Autodesk Inventor part; units mm, degrees
ref_plane "to_ring_F_R_XY" through (20.575, 0, 0) normal (1, 0, 0) x (0, 0, -1)
ref_plane "to_ring_F_R_YZ" through (20.575, 0, 0) normal (0, 0, -1) x (0, 1, 0)
ref_plane "to_ring_F_R_ZX" through (20.575, 0, 0) normal (0, 1, 0) x (1, 0, 0)
sketch "Sketch_1" plane through (0, 0, 0) normal (0, 0, 1) x (1, 0, 0)
  line L0 (23, 0) -> (0, 0)
  line L1 (0, 0) -> (0, 4.5)
  line L2 (0, 4.5) -> (0.5, 5)
  line L3 (0.5, 5) -> (22.5, 5)
  line L4 (22.5, 5) -> (23, 4.5)
  line L5 (23, 4.5) -> (23, 0)
  line L6 (23, 0) -> (0, 0)
revolve "Revolution1" add sketch "Sketch_1" angle 360 about axis through (23, 0, 0) along (1, 0, 0)
sketch "Sketch2" plane through (0, 0, 0) normal (-1, 0, 0) x (0, 0, 1)
  point P0 (0, 0)
hole "Hole1" at (0, 0, 0) direction (1, 0, 0) diameter 4.134 depth 13.8066 tip angle 120 countersink diameter 5 countersink angle 90
sketch "Sketch_20" plane through (0, 0, 0) normal (0, 0, 1) x (1, 0, 0)
  line L0 (23, 0) -> (-23, 0)
  line L1 (20, 9.6) -> (20, 4.8)
  line L2 (20, 4.8) -> (21.15, 4.8)
  line L3 (21.15, 4.8) -> (21.15, 9.6)
  line L4 (21.15, 9.6) -> (20, 9.6)
revolve "Revolution2" cut sketch "Sketch_20" angle 360 about axis through (23, 0, 0) along (1, 0, 0)
ref_plane "to_ring_F_R_XY" through (20.575, 0, 0) normal (1, 0, 0) x (0, 0, -1)
ref_plane "to_ring_F_R_YZ" through (20.575, 0, 0) normal (0, 0, -1) x (0, 1, 0)
ref_plane "to_ring_F_R_ZX" through (20.575, 0, 0) normal (0, 1, 0) x (1, 0, 0)
properties part number "SSFRBF-D10-L23-M5-U3"
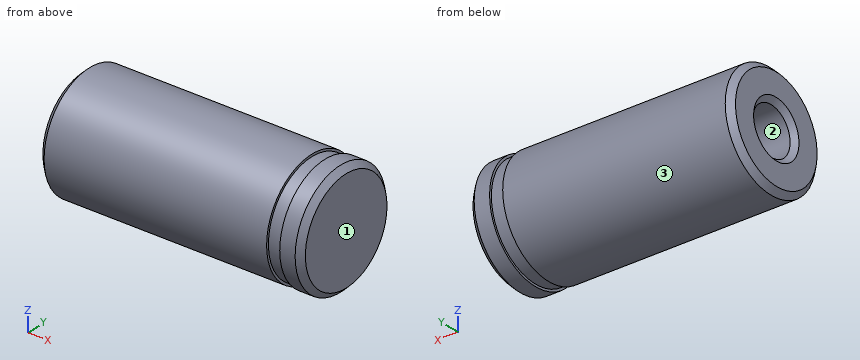
Read the model definition and answer for the solid it produces. Units are mm, in the model's axes. Face numbers are marked on the shaded views. Give positions to 0.01 mm unless a question says otherwise; leave off trailing zeros. Loops run counter-clockwise (first coordinate to the right, second up) from the corner with the lowest first, then second, coordinate; pieces in that order, holes last. Notation, with made-up numbers: (85, 7.25) -> (139, 7.25) arc R10 cw to (139, 13.25) -> close; hole circle Ø10 at (-36.75, 76.5). An arc over 180 degrees is marked (long way). Use a Markdown table: item, result.
Q1. Find the intervals of material crossed by line 1 along Z through (x, y) = (4.25, 0); line 2 along Y through (x, z) = (5.75, 1.75); line 3 along Z through (x, y) = (7.25, 1.25), in increasing order.
Solved:
| item | result |
|---|---|
| line 1 | z = -5 to -2.07, 2.07 to 5 |
| line 2 | y = -4.68 to -1.1, 1.1 to 4.68 |
| line 3 | z = -4.84 to -1.65, 1.65 to 4.84 |
Q2. Section A-A, the plane x = 3 is taken. Determine the outline of the cut face in (y, z), then the cut area to 3 significant figures.
Solved:
| item | result |
|---|---|
| outline | circle Ø10 at (0, 0); hole circle Ø4.13 at (0, 0) |
| area | 65.1 mm^2 |
Q3. Each of these flat-tipped pins is pushed along its axis until it touches: pin 1 (1 mm diameter, centred on x = 5, z = 1, fed in from -Y); pin 2 (1 mm diameter, centred on x = 13.5, y = -3, fed in from +Z); pin 3 (2 mm diameter, centred on y = -0.5, z = -0.5, fed in from -X). Where does it stop, or does it pass through?
Solved:
| item | result |
|---|---|
| pin 1 | stops at y = -4.97 |
| pin 2 | stops at z = 4.33 |
| pin 3 | stops at x = 14.01 |
Q4. Section B-B, the plane x = 14.75 is taken. Determine the outline of the cut face in (y, z), then the cut area to 3 significant figures.
Solved:
| item | result |
|---|---|
| outline | circle Ø10 at (0, 0); hole circle Ø0.87 at (0, 0) |
| area | 78.0 mm^2 |
Q5. Determine the mould class of the marked faces 1, 2 and 3 for opening direction Y: pulls with the +Y half, pulls with the -Y half, needs draft (parallel to the pull), parting line crosses it, or undercut.
Solved:
| item | result |
|---|---|
| face 1 | needs draft |
| face 2 | undercut |
| face 3 | parting line crosses it |
